Geometry check sheet. Reference: drawing and pictorial views, mm from the part's lowest x, y, z. Round coordinates to 2 decimals unless told otherwise and drop trailing zeros. Write each loop counter-clockwise with the first axis right and the second up, starting at its lowest first coordinate (ties: lowest second). Pieces come first, ordered by that corner, then holes. Notation, with made-up numbers: (5.5, 12) - (14.5, 12) arc R14 ccw to (14.5, 27) - close; hole circle Ø3 at (28, 67). An arc over 180 degrees is marked (long way). Return JSON: item names as keys, results as strings.
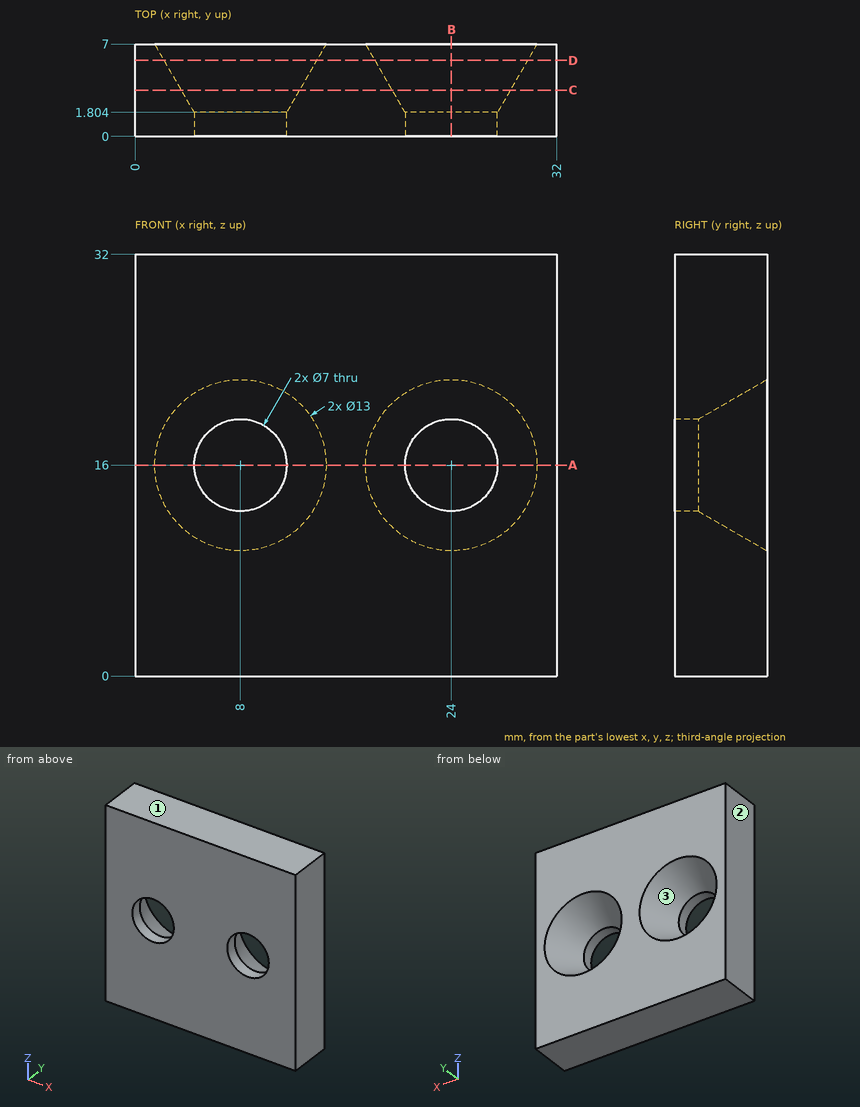
(1) Gauge pin test, flat end, axial feed: pin 1 (2 mm diameter, centred on x = 18, y = 3, fed in from -Z). Record the tip position at first contact, or that the pin passes through.
Response values:
{"pin 1": "stops at z = 0"}
(2) Release check for a two-part mould opening along X. For the marked faces 1, 2 and 3 record: pulls with the +X half, pulls with the -X half, needs draft (parallel to the pull), parting line crosses it, or undercut.
Response values:
{"face 1": "needs draft", "face 2": "pulls with the -X half", "face 3": "undercut"}
(3) Material ranges on line 1 along X through (y, z) = (0.9, 16); line 2 along X through (y, z) = (2, 14); line 3 along Z through (x, y) = (8, 0.95), recorded low to high. Write a range as [from, to].
Response values:
{"line 1": "x = [0, 4.5], [11.5, 20.5], [27.5, 32]", "line 2": "x = [0, 4.99], [11.01, 20.99], [27.01, 32]", "line 3": "z = [0, 12.5], [19.5, 32]"}
(4) Section check B-B, the plane x = 24. Enter the section's corners in (y, z).
Response values:
{"outline": "(0, 0) - (7, 0) - (7, 9.5) - (1.8, 12.5) - (0, 12.5) - close; (0, 19.5) - (1.8, 19.5) - (7, 22.5) - (7, 32) - (0, 32) - close"}
(5) Section check D-D, the plane y = 5.75. Enter the section's corners in (x, z), plus the area to 3 significant figures.
Response values:
{"outline": "(0, 0) - (32, 0) - (32, 32) - (0, 32) - close; hole circle Ø11.56 at (8, 16); hole circle Ø11.56 at (24, 16)", "area": "814 mm^2"}
(6) Section check A-A, the plane z = 16. Enter the section's corners in (x, y).
Response values:
{"outline": "(0, 0) - (4.5, 0) - (4.5, 1.8) - (1.5, 7) - (0, 7) - close; (11.5, 0) - (20.5, 0) - (20.5, 1.8) - (17.5, 7) - (14.5, 7) - (11.5, 1.8) - close; (27.5, 0) - (32, 0) - (32, 7) - (30.5, 7) - (27.5, 1.8) - close"}
(7) Section check C-C, the plane y = 3.5. Enter the section's corners in (x, z).
Response values:
{"outline": "(0, 0) - (32, 0) - (32, 32) - (0, 32) - close; hole circle Ø8.96 at (8, 16); hole circle Ø8.96 at (24, 16)"}
